Input: part model. Units: mm. Frame: model coordinates. Face numbers are marked on the shaded views. Round coordinates to 2 decimals unless told otherwise and drop trailing zeros. Order: outer loops, then holes, each group sorted by start corner. A loop starts at its lowest first (then second) coordinate and runs counter-clockwise, first axis right, second up. Notation, with made-up numbers: (27.5, 15.5) - (37.5, 15.5) arc R24 cw to (37.5, 50.5) - close; hole circle Ø8 at (63, 61.25). An arc over 180 degrees is marked (long way). One line per item, written item: value. Start each with the question number.
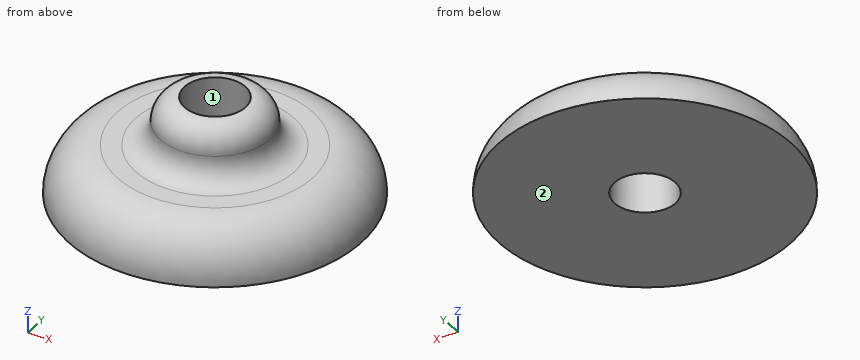
from build123d import *

# Parameters (mm, degrees)
SKETCH1_R           = 6
SKETCH1_R_2         = 1.25
BOSS_EXTRUDE1_DEPTH = 2
SKETCH2_R           = 2.25
SKETCH2_R_2         = 1.25
BOSS_EXTRUDE2_DEPTH = 2
FILLET1_R           = 1
FILLET2_R           = 2


with BuildPart() as part:
    # Sketch1 → Boss-Extrude1 (new body)
    with BuildSketch(Plane.XY):
        Circle(SKETCH1_R)
        Circle(SKETCH1_R_2, mode=Mode.SUBTRACT)
    extrude(amount=BOSS_EXTRUDE1_DEPTH)

    # Sketch2 → Boss-Extrude2 (add)
    with BuildSketch(Plane.XY.offset(2)):
        Circle(SKETCH2_R)
        Circle(SKETCH2_R_2, mode=Mode.SUBTRACT)
    extrude(amount=BOSS_EXTRUDE2_DEPTH)

    # Fillet1
    fillet1_edges = [part.edges().sort_by_distance(p)[0] for p in [
        (-2.25, 0, 4),
        (-2.25, 0, 2),
    ]]
    fillet(fillet1_edges, radius=FILLET1_R - 0.0001)  # a hair under: the kernel refuses the full size

    # Fillet2
    fillet2_edges = [part.edges().sort_by_distance(p)[0] for p in [
        (-6, 0, 2),
    ]]
    fillet(fillet2_edges, radius=FILLET2_R - 0.0001)  # a hair under: the kernel refuses the full size


solid = part.part
Item 1: Pull-direction query (X, two-part tool) for the marked faces 1 and 2; classes: released by +X, released by -X, zero draft, split by the parting line, or undercut.
Item 2: First-contact query: pin 1 Ø4 at (x, y) = (4, -4) entering from +Z; pin 2 Ø1.5 at (y, z) = (-1, 2) entering from -X. Flat tips, straight axial feed; report the tip coordinate or a pass-through.
Item 3: Section query D-D on z = 3.15. Return loops of the section in (x, y).
Item 4: Section query C-C on z = 1.8. Return loops of the section in (x, y).
Item 5: Line query: L1, parallel to Z at x = -0.25, y = -3.75; L2, parallel to Y at x = 0, z = 1.4; L3, parallel to Y at x = 0, z = 2.75. Output: solid intervals per line, ascending.
Geometry results:
1. face 1: undercut
1. face 2: zero draft
2. pin 1: stops at z = 2
2. pin 2: stops at x = -5.48
3. outline: circle Ø4.48 at (0, 0); hole circle Ø2.5 at (0, 0)
4. outline: circle Ø9.74 at (0, 0); hole circle Ø2.5 at (0, 0)
5. L1: z = 0 to 2
5. L2: y = -5.43 to -1.25, 1.25 to 5.43
5. L3: y = -2.28 to -1.25, 1.25 to 2.28
